from build123d import *

# Parameters (mm, degrees)
F0_W     = 50.8
F0_H     = 76.2
F0_W_2   = 44.45
F0_H_2   = 69.85
F2_DEPTH = 1320.8
F3_R     = 3.175


# Not quite as in the source:
# - a variable given as a bare number and used for a length is read in inches; the dataset says mm whatever the document's units were


with BuildPart() as f2:
    # F0 (on Top) → F2 (new body)
    with BuildSketch(Plane.XY):
        Rectangle(F0_W, F0_H)
        Rectangle(F0_W_2, F0_H_2, mode=Mode.SUBTRACT)
    extrude(amount=F2_DEPTH)

    # F3
    f3_edges = [f2.edges().sort_by_distance(p)[0] for p in [
        (25.4, 38.1, 660.4),
        (-25.4, 38.1, 660.4),
        (25.4, -38.1, 660.4),
        (22.225, -34.925, 660.4),
        (-22.225, -34.925, 660.4),
        (-22.225, 34.925, 660.4),
        (22.225, 34.925, 660.4),
        (-25.4, -38.1, 660.4),
    ]]
    fillet(f3_edges, radius=F3_R)


solid = f2.part
Design review of the part built by this model. Coordinates are the model's own, in mm. A direction names the side the tool comes from. Coordinates: 2 decimals unless noted, no trailing zeros. Order: outer loops, then holes, each group sorted by start corner. A loop starts at its lowest first (then second) coordinate and runs counter-clockwise, first axis right, second up. Notation, with made-up numbers: (76.25, -28.75) -> (127.25, -28.75) arc R19 ccw to (127.25, 4.25) -> close; hole circle Ø9 at (27, 52.5). An arc over 180 degrees is marked (long way). Use one line per item in the form item = value. Start each with the question number.
(1) The part is to be moulded in two halves that separate along Y. For faces 1 (the flat face through (-23, 3, 1320.8)), 2 (the flat face through (0, -34.925, 651)), 3 (the flat face through (0, 38.1, 651)), 4 (the flat face through (22.225, 0, 651)), say which applies: +Y half, -Y half, draft (parallel to the pull), parting line (faces both ways), or undercut.
(2) For probe 1 along Y at (x, z) = (-7, 513) (3 decimals); probe 2 along X at (y, z) = (21.5, 1063) (3 decimals); probe 3 along Y at (x, z) = (-20, 1178), list the stretches that pass through material, from the lowest coordinate up.
(3) Add section C-C on z = 115. State the section outline as (x, y) points (3 decimals), plus the area to 3 significant figures.
(4) For faces 5 (the flat face through (-25.4, 0, 651)), 6 (the flat face through (-22.225, 0, 651)), list the 3-axis set-ups (+Z, -Z, +X, -X, +Y, -Y) from which the entire face can be reached by the end or side of a thin tool; tool diameter is ignored.
(5) Add section B-B on x = -7. State the section outline as (y, z) points (3 decimals), plus the area to 3 significant figures.
(6) Add section A-A on y = 0. State the section outline as (x, z) points (3 decimals), plus the area to 3 significant figures.
Answer block:
q1.face_1 = draft
q1.face_2 = undercut
q1.face_3 = +Y half
q1.face_4 = undercut
q2.probe_1 = -38.1 to -34.925, 34.925 to 38.1
q2.probe_2 = -25.4 to -22.225, 22.225 to 25.4
q2.probe_3 = -38.1 to -34.78, 34.78 to 38.1
q3.outline = (-25.4, -34.925) arc R3.175 ccw to (-22.225, -38.1) -> (22.225, -38.1) arc R3.175 ccw to (25.4, -34.925) -> (25.4, 34.925) arc R3.175 ccw to (22.225, 38.1) -> (-22.225, 38.1) arc R3.175 ccw to (-25.4, 34.925) -> close; hole (-22.225, -31.75) arc R3.175 ccw to (-19.05, -34.925) -> (19.05, -34.925) arc R3.175 ccw to (22.225, -31.75) -> (22.225, 31.75) arc R3.175 ccw to (19.05, 34.925) -> (-19.05, 34.925) arc R3.175 ccw to (-22.225, 31.75) -> close
q3.area = 766 mm²
q4.face_5 = +Z, -Z, -X, +Y, -Y
q4.face_6 = +Z, -Z
q5.outline = (-38.1, 0) -> (-34.925, 0) -> (-34.925, 1320.8) -> (-38.1, 1320.8) -> close; (34.925, 0) -> (38.1, 0) -> (38.1, 1320.8) -> (34.925, 1320.8) -> close
q5.area = 8,390 mm²
q6.outline = (-25.4, 0) -> (-22.225, 0) -> (-22.225, 1320.8) -> (-25.4, 1320.8) -> close; (22.225, 0) -> (25.4, 0) -> (25.4, 1320.8) -> (22.225, 1320.8) -> close
q6.area = 8,390 mm²
